Autodesk Inventor part; units mm, degrees
ref_plane "YZ Plane" through (0, 0, 0) normal (1, 0, 0) x (0, 1, 0)
ref_plane "XZ Plane" through (0, 0, 0) normal (0, 1, 0) x (-1, 0, 0)
ref_plane "XY Plane" through (0, 0, 0) normal (0, 0, 1) x (1, 0, 0)
sketch "Sketch1" plane through (0, 0, 0) normal (0, 0, 1) x (1, 0, 0)
  line L0 (-4, 0) -> (4, 0) construction
  line L1 (-4, -4) -> (4, -4)
  line L2 (4, 4) -> (-4, 4)
  arc A0 (-4, 4) -> (-4, -4) centre (-4, 0) ccw
  arc A1 (4, -4) -> (4, 4) centre (4, 0) ccw
  line L3 (-3, 0) -> (3, 0) construction
  line L4 (-3, -3) -> (3, -3)
  line L5 (3, 3) -> (-3, 3)
  arc A2 (-3, 3) -> (-3, -3) centre (-3, 0) ccw
  arc A3 (3, -3) -> (3, 3) centre (3, 0) ccw
  point P0 (0, 0)
extrude "Extrusion1" add sketch "Sketch1" along normal blind 10
sketch "Sketch2" plane through (-4, 4, 0) normal (0, 1, 0) x (1, 0, 0)
  point P0 (4, 0)
  point P1 (4, -5)
hole "Hole1" at (0, 4, 5) direction (0, -1, 0) diameter 3 end through all
properties part number "silicon_tube" material "Rubber, Silicone"
Design review of the part built by this model. Coordinates are the model's own, in mm. A direction names the side the tool comes from. Round coordinates to 2 decimals unless told otherwise and drop trailing zeros. Write each loop counter-clockwise with the first axis right and the second up, starting at its lowest first coordinate (ties: lowest second). Pieces come first, ordered by that corner, then holes. Notation, with made-up numbers: (66.25, 13.25) -> (77.25, 13.25) arc R9 cw to (77.25, 18.25) -> close; hole circle Ø7 at (36, -12.5). An arc over 180 degrees is marked (long way). One line per item, written item: value. Start each with the question number.
Q1. The part is to be moulded in two halves that separate along Z. For faces 1 (the face through (-0.1, -3.5, 0)), 2 (the face through (0.575, -3.507, 6.386)), 3 (the face through (2, 4, 5)), say which applies: pulls with the +Z half, pulls with the -Z half, needs draft (parallel to the pull), parting line crosses it, or undercut.
Q2. Add section B-B (y = 2.25). Give the boundary of the cut face in (x, z).
Q3. To check wall thickness, follow probe 1 along Y at (x, z) = (1.75, 6.5); probe 2 along Z at (x, y) = (0, 3.7); probe 3 along X at (y, z) = (0, 7.5). State the ranges of each line that lie inside material, in increasing order.
Q4. Add section A-A (x = 2.5). Give the boundary of the cut face in (y, z).
Q5. Tool access review of faces 4 (the face through (1.3, -3, 3.8)), 5 (the face through (-0.1, -3.5, 10)): name each direction out of +Z, -Z, +X, -X, +Y, -Y from which nothing blocks a thin tool from reaching the whole face with its end or side.
Q6. Insertion check: P1, Ø2.5, axis at x = 0, z = 5, coming from the -Y side. The pin has a flat end and moves straight along its axis. Give the tip position at first contact, or say it passes through.
Q7. Add section C-C (z = 4.75). Give the boundary of the cut face in (x, y).
Q8. Add section D-D (x = 0.75). Give the boundary of the cut face in (y, z).
Response:
1. face 1: pulls with the -Z half
1. face 2: undercut
1. face 3: needs draft
2. outline: (-7.31, 0) -> (-4.98, 0) -> (-4.98, 10) -> (-7.31, 10) -> close; (4.98, 0) -> (7.31, 0) -> (7.31, 10) -> (4.98, 10) -> close
3. probe 1: y = -4 to -3, 3 to 4
3. probe 2: z = 0 to 3.5, 6.5 to 10
3. probe 3: x = -8 to -6, 6 to 8
4. outline: (-4, 0) -> (-3, 0) -> (-3, 10) -> (-4, 10) -> close; (3, 0) -> (4, 0) -> (4, 10) -> (3, 10) -> close
5. face 4: +Z, -Z
5. face 5: +Z, +X, -X, +Y, -Y
6. P1: passes through
7. outline: (-4, -4) -> (-1.48, -4) -> (-1.48, -3) -> (-3, -3) arc R3 cw to (-3, 3) -> (-1.48, 3) -> (-1.48, 4) -> (-4, 4) arc R4 ccw to start; (1.48, -4) -> (4, -4) arc R4 ccw to (4, 4) -> (1.48, 4) -> (1.48, 3) -> (3, 3) arc R3 cw to (3, -3) -> (1.48, -3) -> close
8. outline: (-4, 0) -> (-3, 0) -> (-3, 3.7) -> (-4, 3.7) -> close; (-4, 6.3) -> (-3, 6.3) -> (-3, 10) -> (-4, 10) -> close; (3, 0) -> (4, 0) -> (4, 3.7) -> (3, 3.7) -> close; (3, 6.3) -> (4, 6.3) -> (4, 10) -> (3, 10) -> close
